The model under review builds one solid part; all positions refer to its coordinate system, in mm. A direction names the side the tool comes from. Give positions to 0.01 mm unless a question says otherwise; leave off trailing zeros. Write each loop counter-clockwise with the first axis right and the second up, starting at its lowest first coordinate (ties: lowest second). Pieces come first, ordered by that corner, then holes. Notation, with made-up numbers: M -11,63 L 24,63 A23 ccw 24,102 Z; hole C -24.75,79 d4. An arc over 180 degrees is marked long. Write item = value, one per line. Start each with the question number.
```python
from build123d import *

# Parameters (mm, degrees)
F0_W     = 205
F0_H     = 285
F1_DEPTH = 3
F2_W     = 205
F2_H     = 285
F2_W_2   = 98
F2_H_2   = 178
F3_DEPTH = 50


with BuildPart() as f1:
    # F0 (on Top) → F1 (new body)
    with BuildSketch(Plane.XY):
        Rectangle(F0_W, F0_H)
    extrude(amount=F1_DEPTH)

    # F2 (on face) → F3 (join)
    with BuildSketch(Plane.XY.offset(3)):
        Rectangle(F2_W, F2_H)
        with Locations((-50.5, -50.5)):
            Rectangle(F2_W_2, F2_H_2, mode=Mode.SUBTRACT)
        with Locations((50.5, -50.5)):
            Rectangle(F2_W_2, F2_H_2, mode=Mode.SUBTRACT)
        Polygon((-99.5, 139.5), (99.5, 139.5), (99.5, 41.5), (0, 41.5), (-99.5, 41.5), align=None, mode=Mode.SUBTRACT)
    extrude(amount=F3_DEPTH)


solid = f1.part
```
Item 1: We need section D-D, the plane y = 96.5. Write out the cut boundary in (x, z).
Item 2: The part is to be moulded in two halves that separate along X. For faces 3 (the flat face through (1.5, -52, 28)), 4 (the flat face through (-1, 142.5, 26)), 5 (the flat face through (-102.5, -2, 26)), say which applies: released by +X, released by -X, zero draft, split by the parting line, or undercut.
Item 3: For faces 1 (the flat face through (-1, -142.5, 26)), 2 (the flat face through (-51, -49, 3)), list the 3-axis set-ups (+Z, -Z, +X, -X, +Y, -Y) from which the entire face can be reached by the end or side of a thin tool; tool diameter is ignored.
Item 4: We need section C-C, the plane x = 76. Write out the cut boundary in (y, z).
Item 5: To check wall thickness, follow probe 1 along Y at (x, z) = (-40, 38); probe 2 along X at (y, z) = (-114, 4.5); probe 3 along Z at (x, y) = (-66.5, 69.5). State the ranges of each line that lie inside material, in increasing order. Write a range as [from, to].
Item 6: We need section B-B, the plane z = 19. Write out the cut boundary in (x, y), and give its area (4 significant figures).
Item 7: We need section A-A, the plane y = -65.5. Write out the cut boundary in (x, z), and give its area (4 significant figures).
Item 8: Clearance check with flat-ended pins moving along their axes: P1, Ø3, axis at x = -67.5, y = -76, coming from the +Z side; P2, Ø3, axis at x = 68.5, y = 23, coming from the -Z side. State where each tip first meets the part, or that it passes through.
Worked out:
q1.outline = M -102.5,0 L 102.5,0 L 102.5,53 L 99.5,53 L 99.5,3 L -99.5,3 L -99.5,53 L -102.5,53 Z
q2.face_3 = undercut
q2.face_4 = zero draft
q2.face_5 = released by -X
q3.face_1 = +Z, -Z, +X, -X, -Y
q3.face_2 = +Z
q4.outline = M -142.5,0 L 142.5,0 L 142.5,53 L 139.5,53 L 139.5,3 L 41.5,3 L 41.5,53 L 38.5,53 L 38.5,3 L -139.5,3 L -139.5,53 L -142.5,53 Z
q5.probe_1 = [-142.5, -139.5], [38.5, 41.5], [139.5, 142.5]
q5.probe_2 = [-102.5, -99.5], [-1.5, 1.5], [99.5, 102.5]
q5.probe_3 = [0, 3]
q6.outline = M -102.5,-142.5 L 102.5,-142.5 L 102.5,142.5 L -102.5,142.5 Z; hole M -99.5,-139.5 L -1.5,-139.5 L -1.5,38.5 L -99.5,38.5 Z; hole M -99.5,41.5 L 99.5,41.5 L 99.5,139.5 L -99.5,139.5 Z; hole M 1.5,-139.5 L 99.5,-139.5 L 99.5,38.5 L 1.5,38.5 Z
q6.area = 4,035 mm²
q7.outline = M -102.5,0 L 102.5,0 L 102.5,53 L 99.5,53 L 99.5,3 L 1.5,3 L 1.5,53 L -1.5,53 L -1.5,3 L -99.5,3 L -99.5,53 L -102.5,53 Z
q7.area = 1,065 mm²
q8.P1 = 3
q8.P2 = 0
